from build123d import *

# Parameters (mm, degrees)
SKETCH1_W           = 300
SKETCH1_H           = 50
BOSS_EXTRUDE1_DEPTH = 60
SKETCH5_W           = 22.63
SKETCH5_H           = 12.19
CUT_EXTRUDE2_DEPTH  = 12.84
SKETCH4_W           = 20
SKETCH4_H           = 6
CUT_EXTRUDE3_DEPTH  = 2


with BuildPart() as part:
    # Sketch1 → Boss-Extrude1 (new body)
    with BuildSketch(Plane.XY):
        with Locations((150, -25)):
            Rectangle(SKETCH1_W, SKETCH1_H)
    extrude(amount=BOSS_EXTRUDE1_DEPTH)

    # Sketch5 → Cut-Extrude2 (cut)
    with BuildSketch(Plane.XY.offset(60)):
        with Locations((11.315, -25.468667548)):
            Rectangle(SKETCH5_W, SKETCH5_H)
    extrude(amount=-CUT_EXTRUDE2_DEPTH, mode=Mode.SUBTRACT)

    # Sketch4 → Cut-Extrude3 (cut)
    with BuildSketch(Plane.XY.offset(60)):
        with Locations((275.959149907, -22.479653517)):
            Rectangle(SKETCH4_W, SKETCH4_H)
    extrude(amount=-CUT_EXTRUDE3_DEPTH, mode=Mode.SUBTRACT)


solid = part.part
Work out the finished part from the listing and answer in its coordinate system (mm). A direction names the side the tool comes from. Round coordinates to 2 decimals unless told otherwise and drop trailing zeros. Write each loop counter-clockwise with the first axis right and the second up, starting at its lowest first coordinate (ties: lowest second). Pieces come first, ordered by that corner, then holes. Notation, with made-up numbers: (24, 35.25) - (63, 35.25) arc R30 ccw to (63, 70.25) - close; hole circle Ø4 at (-37, 32). An arc over 180 degrees is marked (long way). Answer in a Markdown table with one row per item. Add a question column.
1. The mould has two halves that part along Y. Classify faces 1 (the flat face through (148, -50, 30)), 2 (the flat face through (276, -22, 58)), 3 (the flat face through (148, -25, 0)): +Y half, -Y half, draft (parallel to the pull), parting line (faces both ways), or undercut.
2. Given pin 1 (1.6 mm diameter, centred on y = -21.5, z = 59, fed in from -X); pin 2 (10 mm diameter, centred on x = 8.5, y = -25, fed in from +Z), each flat-ended and moving along its own axis, determine where each tip first touches the part or whether it passes through.
3. For faces 4 (the flat face through (11, -31.564, 54)), 5 (the flat face through (148, 0, 30)), determine the directions among +Z, -Z, +X, -X, +Y, -Y from which every point of the face is accessible in a straight line to the end or side of a thin tool.
4. A cutting plane is placed at A-A, the plane z = 55. Determine the outline of the cut face in (x, y).
Worked out:
| question | item | result |
|---|---|---|
| 1 | face 1 | -Y half |
| 1 | face 2 | undercut |
| 1 | face 3 | draft |
| 2 | pin 1 | x = 22.63 |
| 2 | pin 2 | z = 47.16 |
| 3 | face 4 | +Z, -X |
| 3 | face 5 | +Z, -Z, +X, -X, +Y |
| 4 | outline | (0, -50) - (300, -50) - (300, 0) - (0, 0) - (0, -19.37) - (22.63, -19.37) - (22.63, -31.56) - (0, -31.56) - close |
